from build123d import *

# Parameters (mm, degrees)
F0_W     = 193.675
F0_H     = 110.49
F1_DEPTH = 38.1
F2_R     = 3.175
F3_T     = -2.54


with BuildPart() as f1:
    # F0 (on Top) → F1 (new body)
    with BuildSketch(Plane.XY):
        with Locations((-19.322108, 8.169052)):
            Rectangle(F0_W, F0_H)
    extrude(amount=F1_DEPTH)

    # F2
    f2_edges = [f1.edges().sort_by_distance(p)[0] for p in [
        (-116.159608, 8.169052, 38.1),
        (-19.322108, 63.414052, 38.1),
        (-19.322108, -47.075948, 38.1),
        (77.515392, 8.169052, 38.1),
        (77.515392, 63.414052, 19.05),
        (77.515392, -47.075948, 19.05),
        (-116.159608, -47.075948, 19.05),
        (-116.159608, 63.414052, 19.05),
    ]]
    fillet(f2_edges, radius=F2_R)

    # F3
    f3_openings = [f1.faces().sort_by_distance(p)[0] for p in [
        (-19.322108, 8.169052, 0),
    ]]
    offset(amount=F3_T, openings=f3_openings)


solid = f1.part
Read the model definition and answer for the solid it produces. Units are mm, in the model's axes. A direction names the side the tool comes from. Give positions to 0.01 mm unless a question says otherwise; leave off trailing zeros. Write each loop counter-clockwise with the first axis right and the second up, starting at its lowest first coordinate (ties: lowest second). Pieces come first, ordered by that corner, then holes. Notation, with made-up numbers: (78, -36) - (117, -36) arc R21 cw to (117, -24) - close; hole circle Ø3 at (30, 12.5). An arc over 180 degrees is marked (long way). Return JSON: item names as keys, results as strings.
Q1. Consider line 1 along X through (y, z) = (-24.5, 27); line 2 along Y through (x, z) = (-7, 34); line 3 along Z through (x, y) = (-100, -24.5). Determine where each line is inside the solid, lowest interval first. Write a range as [from, to].
Reply:
{"line 1": "[-116.16, -113.62], [74.98, 77.52]", "line 2": "[-47.08, -44.54], [60.87, 63.41]", "line 3": "[35.56, 38.1]"}
Q2. For a pull along X with two mould halves and no side action, classify faces 3 (the face through (-20, 62, 0)), 4 (the face through (74.975, 7, 17)), 5 (the face through (77.515, 7, 17)), 6 (the face through (-21, 60.874, 17)) as released by +X, released by -X, zero draft, split by the parting line, or undercut.
Reply:
{"face 3": "zero draft", "face 4": "undercut", "face 5": "released by +X", "face 6": "undercut"}
Q3. A cutting plane is placed at C-C, the plane y = 12.5. Determine the outline of the cut face in (x, z) (3 decimals).
Reply:
{"outline": "(-116.16, 0) - (-113.62, 0) - (-113.62, 34.925) arc R0.635 cw to (-112.985, 35.56) - (74.34, 35.56) arc R0.635 cw to (74.975, 34.925) - (74.975, 0) - (77.515, 0) - (77.515, 34.925) arc R3.175 ccw to (74.34, 38.1) - (-112.985, 38.1) arc R3.175 ccw to (-116.16, 34.925) - close"}
Q4. A cutting plane is placed at B-B, the plane x = -50.5. Determine the outline of the cut face in (y, z) (3 decimals), and give its area (3 significant figures).
Reply:
{"outline": "(-47.076, 0) - (-44.536, 0) - (-44.536, 34.925) arc R0.635 cw to (-43.901, 35.56) - (60.239, 35.56) arc R0.635 cw to (60.874, 34.925) - (60.874, 0) - (63.414, 0) - (63.414, 34.925) arc R3.175 ccw to (60.239, 38.1) - (-43.901, 38.1) arc R3.175 ccw to (-47.076, 34.925) - close", "area": "457 mm²"}
Q5. A cutting plane is placed at A-A, the plane z = 25. Determine the outline of the cut face in (x, y) (3 decimals).
Reply:
{"outline": "(-116.16, -43.901) arc R3.175 ccw to (-112.985, -47.076) - (74.34, -47.076) arc R3.175 ccw to (77.515, -43.901) - (77.515, 60.239) arc R3.175 ccw to (74.34, 63.414) - (-112.985, 63.414) arc R3.175 ccw to (-116.16, 60.239) - close; hole (-113.62, -43.901) arc R0.635 ccw to (-112.985, -44.536) - (74.34, -44.536) arc R0.635 ccw to (74.975, -43.901) - (74.975, 60.239) arc R0.635 ccw to (74.34, 60.874) - (-112.985, 60.874) arc R0.635 ccw to (-113.62, 60.239) - close"}
Q6. For faces 1 (the face through (-21, -44.536, 17)), 2 (the face through (-21, -47.076, 17)), determine the directions among +Z, -Z, +X, -X, +Y, -Y from which every point of the face is accessible in a straight line to the end or side of a thin tool.
Reply:
{"face 1": "-Z", "face 2": "+Z, -Z, +X, -X, -Y"}
